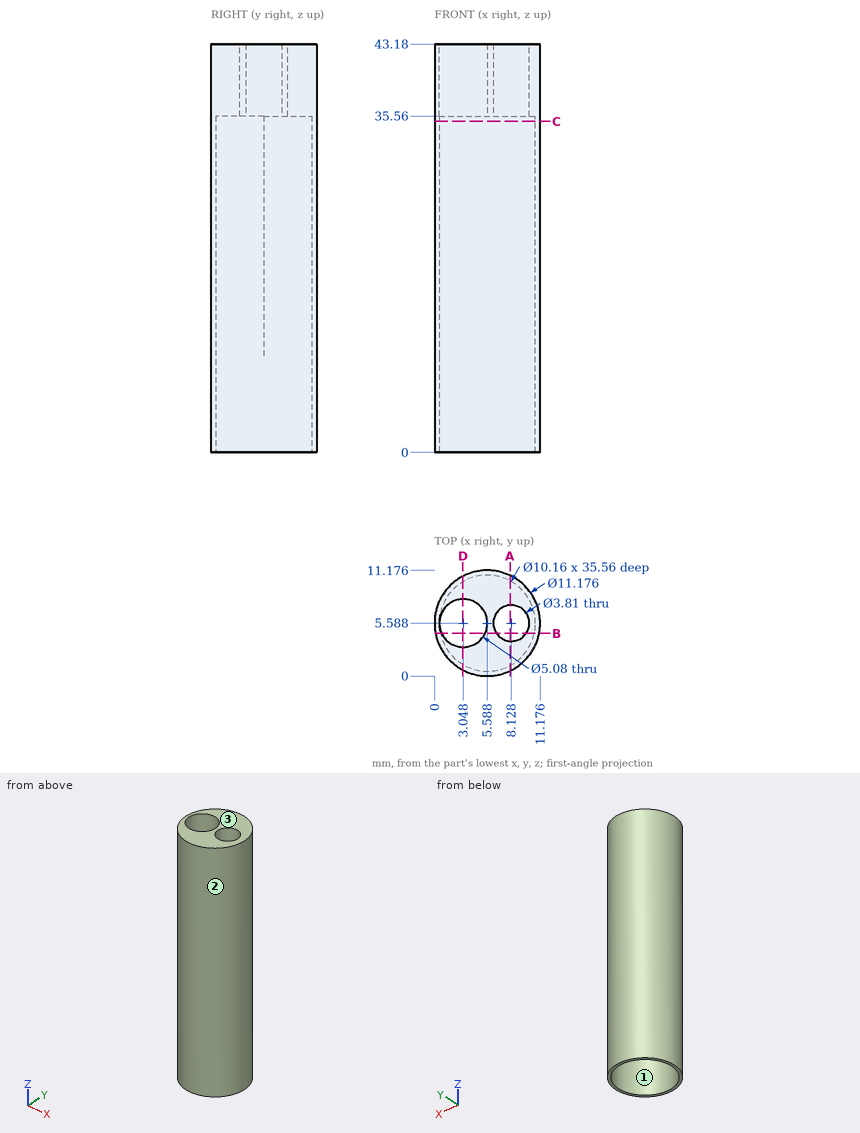
Answer from the drawing. Dimensions are ordinates in mm from the lowest x, y and z of the part. Give positions to 0.01 mm unless a question says otherwise; leave off trailing zeros. Order: outer loops, then holes, each group sorted by start corner. A loop starts at its lowest first (then second) coordinate and runs counter-clockwise, first axis right, second up.
(1) Find section C-C (z = 35). Give the vertices of the cut face in (x, y), plus the area to 3 significant figures.
(2) Find section D-D (x = 3). Give the vertices of the cut face in (y, z), plus the area to 3 significant figures.
(3) Find section A-A (x = 8). Give the vertices of the cut face in (y, z), plus the area to 3 significant figures.
(4) Straight lines are drawn through the part: L1, parallel to Y at x = 8.5, z = 39.5; L2, parallel to X at y = 7.25, z = 10; L3, parallel to X at y = 7.5, z = 30. For each, find the intervals that lie inside material, in ascending order.
(5) For a pull along Y with two mould halves and no side action, classify the marked faces 1, 2 and 3 as released by +Y, released by -Y, zero draft, split by the parting line, or undercut.
(6) Given pin 1 (4 mm diameter, centred on y = 1.5, z = 9.5, fed in from +X); pin 2 (6 mm diameter, centred on x = 5.588, y = 5.588, fed in from -Z); pin 3 (5 mm diameter, centred on x = 8.5, z = 11.5, fed in from +Y), each flat-ended and moving along its own axis, determine where each tip first touches the part or whether it passes through.
(7) Find section B-B (y = 4.5). Give the vertices of the cut face in (x, z), plus the area to 3 significant figures.
Result sheet:
1. outline: circle Ø11.18 at (5.59, 5.59); hole circle Ø10.16 at (5.59, 5.59)
1. area: 17.0 mm2
2. outline: (0.64, 0) - (1.22, 0) - (1.22, 35.56) - (3.05, 35.56) - (3.05, 43.18) - (0.64, 43.18) - close; (8.13, 35.56) - (9.96, 35.56) - (9.96, 0) - (10.54, 0) - (10.54, 43.18) - (8.13, 43.18) - close
2. area: 78.1 mm2
3. outline: (0.55, 0) - (1.12, 0) - (1.12, 35.56) - (3.69, 35.56) - (3.69, 43.18) - (0.55, 43.18) - close; (7.49, 35.56) - (10.06, 35.56) - (10.06, 0) - (10.63, 0) - (10.63, 43.18) - (7.49, 43.18) - close
3. area: 88.4 mm2
4. L1: y = 0.82 to 3.72, 7.46 to 10.36
4. L2: x = 0.25 to 0.79, 10.39 to 10.92
4. L3: x = 0.34 to 0.88, 10.29 to 10.84
5. face 1: undercut
5. face 2: split by the parting line
5. face 3: zero draft
6. pin 1: stops at x = 10.77
6. pin 2: stops at z = 35.56
6. pin 3: stops at y = 11.16
7. outline: (0.11, 0) - (0.63, 0) - (0.63, 35.56) - (0.75, 35.56) - (0.75, 43.18) - (0.11, 43.18) - close; (5.34, 35.56) - (6.56, 35.56) - (6.56, 43.18) - (5.34, 43.18) - close; (9.69, 35.56) - (10.55, 35.56) - (10.55, 0) - (11.07, 0) - (11.07, 43.18) - (9.69, 43.18) - close
7. area: 61.6 mm2
